Work out the finished part from the listing and answer in its coordinate system (mm). A direction names the side the tool comes from. Coordinates: 2 decimals unless noted, no trailing zeros. Order: outer loops, then holes, each group sorted by start corner. A loop starts at its lowest first (then second) coordinate and runs counter-clockwise, first axis right, second up.
1. Determine the mould class of faces 1 (the flat face through (0, 0, 0)), 2 (the flat face through (-25, 0, 4)), 3 (the flat face through (0, 0, 2)) for opening direction X: +X half, -X half, draft (parallel to the pull), parting line (faces both ways), or undercut.
2. A tool of negligible diameter and unlimited length cuts with its end or side. For faces 4 (the flat face through (20, 0, 7.2)), 5 (the flat face through (-18.28, -0.13, 4.64)), from which of +Z, -Z, +X, -X, +Y, -Y can it reach the whole face along a straight path? Write none if from no direction.
3. Find the intervals of material crossed by probe 1 along Z at (x, y) = (12, -6.5); probe 2 along Z at (x, y) = (17, 7.25); probe 3 along X at (y, z) = (0, 6.5), in increasing order.
4. The part is cut by section A-A, the plane z = 6.75. Give the vertices of the cut face in (x, y).
5. The part is cut by section C-C, the plane x = -8.5. Give the vertices of the cut face in (y, z), then the cut area to 3 significant figures.
6. The part is cut by section B-B, the plane y = 3. Give the vertices of the cut face in (x, z).
7. A flat-ended cylindrical pin translates along its axis: pin 1 Ø5.5 at (x, y) = (5.5, -1) entering from +Z. Find the tip coordinate at first contact, or state that the pin passes through.
Autodesk Fusion 360 part; units mm, degrees
ref_plane "工作平面1" through (0, 0, 0) normal (0, 0, 1) x (1, 0, 0)
sketch "草图1" plane through (0, 0, 0) normal (0, 0, 1) x (1, 0, 0)
  line L0 (-25, -9) -> (25, -9)
  line L1 (25, -9) -> (25, 9)
  line L2 (25, 9) -> (-25, 9)
  line L3 (-25, 9) -> (-25, -9)
extrude "Coupon base" add sketch "草图1" along normal blind 2
ref_plane "工作平面2" through (0, 0, 2) normal (0, 0, 1) x (1, 0, 0)
sketch "草图2" plane through (0, 0, 2) normal (0, 0, 1) x (1, 0, 0)
  line L0 (-25, -9) -> (-20.39, -9)
  line L1 (-20.39, -9) -> (-20.39, 9)
  line L2 (-20.39, 9) -> (-25, 9)
  line L3 (-25, 9) -> (-25, -9)
ref_plane "工作平面3" through (0, 0, 7.2) normal (0, 0, 1) x (1, 0, 0)
sketch "草图3" plane through (0, 0, 7.2) normal (0, 0, 1) x (1, 0, 0)
  line L0 (-25, -9) -> (-16.23, -9)
  line L1 (-16.23, -9) -> (-16.23, 9)
  line L2 (-16.23, 9) -> (-25, 9)
  line L3 (-25, 9) -> (-25, -9)
loft "Coupon dovetail rail" add profiles "草图2", "草图3" section 1 section 2
ref_plane "工作平面4" through (0, 0, 2) normal (0, 0, 1) x (1, 0, 0)
sketch "草图4" plane through (0, 0, 2) normal (0, 0, 1) x (1, 0, 0)
  line L0 (20.39, -9) -> (25, -9)
  line L1 (25, -9) -> (25, 9)
  line L2 (25, 9) -> (20.39, 9)
  line L3 (20.39, 9) -> (20.39, -9)
ref_plane "工作平面5" through (0, 0, 7.2) normal (0, 0, 1) x (1, 0, 0)
sketch "草图5" plane through (0, 0, 7.2) normal (0, 0, 1) x (1, 0, 0)
  line L0 (16.23, -9) -> (25, -9)
  line L1 (25, -9) -> (25, 9)
  line L2 (25, 9) -> (16.23, 9)
  line L3 (16.23, 9) -> (16.23, -9)
loft "Coupon dovetail rail (1)" add profiles "草图4", "草图5" section 1 section 2
Geometry says:
1. face 1: draft
1. face 2: -X half
1. face 3: undercut
2. face 4: +Z, +X, -X, +Y, -Y
2. face 5: +Y, -Y
3. probe 1: z = 0 to 2
3. probe 2: z = 0 to 2, 6.24 to 7.2
3. probe 3: x = -25 to -16.79, 16.79 to 25
4. outline: (-25, -9) - (-16.59, -9) - (-16.59, 9) - (-25, 9) - close; (16.59, -9) - (25, -9) - (25, 9) - (16.59, 9) - close
5. outline: (-9, 0) - (9, 0) - (9, 2) - (-9, 2) - close
5. area: 36.0 mm2
6. outline: (-25, 0) - (25, 0) - (25, 7.2) - (16.23, 7.2) - (20.39, 2) - (-20.39, 2) - (-16.23, 7.2) - (-25, 7.2) - close
7. pin 1: stops at z = 2
